Autodesk Inventor part; units mm, degrees
ref_plane "Work Plane1" through (29, -49.6, 0) normal (0, -1, 0) x (1, 0, 0)
ref_plane "YZ Plane" through (0, 0, 0) normal (1, 0, 0) x (0, 1, 0)
ref_plane "XZ Plane" through (0, 0, 0) normal (0, 1, 0) x (-1, 0, 0)
sketch "Sketch2" plane through (0, 0, 0) normal (0, 0, 1) x (1, 0, 0)
  line L0 (29, -124.2) -> (29, -103.2)
  line L1 (29, -103.2) -> (25, -103.2)
  line L2 (25, -103.2) -> (25, -63.2)
  line L3 (25, -63.2) -> (29, -63.2)
  line L4 (29, -63.2) -> (29, -36)
  line L5 (29, -36) -> (25, -36)
  line L6 (25, -36) -> (25, 4)
  line L7 (25, 4) -> (29, 4)
  line L8 (29, 4) -> (29, 25)
  line L9 (29, 29) -> (29, 25)
  line L10 (29, 25) -> (69, 25)
  line L11 (29, -128.2) -> (29, -124.2)
  line L12 (29, -124.2) -> (69, -124.2)
  line L13 (49, -124.2) -> (49, -141.5735)
  line L14 (73, 4) -> (69, 4)
  line L15 (73, -36) -> (73, 4)
  line L16 (69, -36) -> (73, -36)
  line L17 (73, -63.2) -> (69, -63.2)
  line L18 (73, -103.2) -> (73, -63.2)
  line L19 (69, -103.2) -> (73, -103.2)
  line L20 (69, -103.2) -> (69, -124.2)
  line L21 (69, 25) -> (69, 4)
  line L22 (69, -36) -> (69, -63.2)
  point P0 (0, 0)
  dimension "d15" = 4
  dimension "d16" = 40
  dimension "d17" = 4
  dimension "d20" = 40
  dimension "d21" = 40
  dimension "d22" = 149.2
extrude "Extrusion3" add sketch "Sketch2" along normal blind 4
sketch "Sketch3" plane through (0, 0, 4) normal (0, 0, 1) x (1, 0, 0)
  line L0 (29, -103.2) -> (29, -124.2)
  line L1 (29, -124.2) -> (69, -124.2)
  line L2 (69, -124.2) -> (69, -103.2)
  line L3 (69, -103.2) -> (73, -103.2)
  line L4 (73, -103.2) -> (73, -63.2)
  line L5 (73, -63.2) -> (69, -63.2)
  line L6 (69, -63.2) -> (69, -36)
  line L7 (69, -36) -> (73, -36)
  line L8 (73, -36) -> (73, 4)
  line L9 (73, 4) -> (69, 4)
  line L10 (69, 4) -> (69, 25)
  line L11 (69, 25) -> (29, 25)
  line L12 (29, 25) -> (29, 4)
  line L13 (29, 4) -> (25, 4)
  line L14 (25, 4) -> (25, -36)
  line L15 (25, -36) -> (29, -36)
  line L16 (29, -36) -> (29, -63.2)
  line L17 (29, -63.2) -> (25, -63.2)
  line L18 (25, -63.2) -> (25, -103.2)
  line L19 (25, -103.2) -> (29, -103.2)
  line L20 (54, 29) -> (44, 29)
  line L21 (44, 29) -> (44, 25)
  line L22 (44, 25) -> (54, 25)
  line L23 (54, 25) -> (54, 29)
  point P0 (0, 0)
  point P1 (49, 25)
  dimension "d23" = 10
  dimension "d24" = 4
extrude "Extrusion4" add sketch "Sketch3" against normal blind 4 contours L21 L20 L23 L11
ref_plane "Work Plane1" through (29, -49.6, 0) normal (0, -1, 0) x (1, 0, 0)
mirror "Mirror1" about plane through (29, -49.6, 0) normal (0, -1, 0) of "Extrusion4"
equation "\"d23\" = D"
equation "\"D\" = 10"
properties part number "F2"
For this review, take the finished solid that the model builds, in its own axes (mm). A direction names the side the tool comes from. Give positions to 0.01 mm unless a question says otherwise; leave off trailing zeros. Order: outer loops, then holes, each group sorted by start corner. A loop starts at its lowest first (then second) coordinate and runs counter-clockwise, first axis right, second up.
1) Wall thickness on line 1 (Y direction, x = 40, z = 2.5); line 2 (X direction, y = -36.5, z = 1.8); line 3 (Y direction, x = 69.5, z = 0.35): over which ranges is each line inside the solid? List them lowest first.
2) Insertion check: pin 1 (2 mm diameter, centred on y = 28, z = 3, fed in from +X); pin 2 (1.2 mm diameter, centred on x = 70, z = 1.5, fed in from -Y); pin 3 (1 mm diameter, centred on x = 36, z = 3, fed in from +Y). Each pin has a flat end and moves straight along its axis. Give the tip position at first contact, or say it passes through.
3) Take a section at B-B (y = 19.5). Give the boundary of the cut face in (x, z), then the cut area to 3 significant figures.
4) The part is to be moulded in two halves that separate along Y. For faces 1 (the face through (71, -63.2, 2)), 2 (the face through (27, 4, 2)), 3 (the face through (36, -124.2, 2)), 4 (the face through (29, 14, 2)), say which applies: released by +Y, released by -Y, zero draft, split by the parting line, or undercut.
5) Take a section at C-C (x = 40). Give the boundary of the cut face in (y, z).
6) For faces 5 (the face through (71, -36, 2)), 6 (the face through (27, -63.2, 2)), 7 (the face through (71, 4, 2)), 8 (the face through (44, 27, 2)), 9 (the face through (54, -126, 2)), list the 3-axis set-ups (+Z, -Z, +X, -X, +Y, -Y) from which the entire face can be reached by the end or side of a thin tool; tool diameter is ignored.
7) Take a section at A-A (z = 1.4). Give the boundary of the cut face in (x, y), then the cut area to 3 significant figures.
Derived:
1. line 1: y = -124.2 to 25
1. line 2: x = 29 to 69
1. line 3: y = -103.2 to -63.2, -36 to 4
2. pin 1: stops at x = 54
2. pin 2: stops at y = -103.2
2. pin 3: stops at y = 25
3. outline: (29, 0) - (69, 0) - (69, 4) - (29, 4) - close
3. area: 160 mm2
4. face 1: undercut
4. face 2: released by +Y
4. face 3: released by -Y
4. face 4: zero draft
5. outline: (-124.2, 0) - (25, 0) - (25, 4) - (-124.2, 4) - close
6. face 5: +Z, -Z, +X
6. face 6: +Z, -Z, -X
6. face 7: +Z, -Z, +X, +Y
6. face 8: +Z, -Z, -X, +Y
6. face 9: +Z, -Z, +X, -Y
7. outline: (25, -103.2) - (29, -103.2) - (29, -124.2) - (44, -124.2) - (44, -128.2) - (54, -128.2) - (54, -124.2) - (69, -124.2) - (69, -103.2) - (73, -103.2) - (73, -63.2) - (69, -63.2) - (69, -36) - (73, -36) - (73, 4) - (69, 4) - (69, 25) - (54, 25) - (54, 29) - (44, 29) - (44, 25) - (29, 25) - (29, 4) - (25, 4) - (25, -36) - (29, -36) - (29, -63.2) - (25, -63.2) - close
7. area: 6,690 mm2
